```python
from build123d import *

# Parameters (mm, degrees)
F1_DEPTH = 16


with BuildPart() as f1:
    # F0 (on Top) → F1 (new body)
    with BuildSketch(Plane.XY):
        Polygon((0.414211, 0.041402), (-1.415181, 0.041402), (-1.411876, 0), (-0.781621, 0), (-0.497795, -0.270558), (0.132981, -0.270558), (0.417517, 0), align=None)
        Polygon((0.420945, 0.041402), (0.414211, 0.041402), (0.417517, 0), align=None)
        Polygon((2.243604, 0.041402), (0.420945, 0.041402), (0.417517, 0), (1.047772, 0), (1.331597, -0.270558), (1.962374, -0.270558), (2.246909, 0), align=None)
        Polygon((2.250337, 0.041402), (2.243604, 0.041402), (2.246909, 0), align=None)
        Polygon((4.072996, 0.041402), (2.250337, 0.041402), (2.246909, 0), (2.877164, 0), (3.160989, -0.270558), (3.791766, -0.270558), (4.076301, 0), align=None)
        Polygon((4.079729, 0.041402), (4.072996, 0.041402), (4.076301, 0), align=None)
        Polygon((5.902388, 0.041402), (4.079729, 0.041402), (4.076301, 0), (4.706556, 0), (4.990381, -0.270558), (5.621158, -0.270558), (5.905694, 0), align=None)
        Polygon((5.909122, 0.041402), (5.902388, 0.041402), (5.905694, 0), align=None)
        Polygon((7.73178, 0.041402), (5.909122, 0.041402), (5.905694, 0), (6.535948, 0), (6.819774, -0.270558), (7.450551, -0.270558), (7.735086, 0), align=None)
        Polygon((7.738514, 0.041402), (7.73178, 0.041402), (7.735086, 0), align=None)
        Polygon((9.561173, 0.041402), (7.738514, 0.041402), (7.735086, 0), (8.365341, 0), (8.649166, -0.270558), (9.279943, -0.270558), (9.564478, 0), align=None)
        Polygon((9.567906, 0.041402), (9.561173, 0.041402), (9.564478, 0), align=None)
        Polygon((11.390565, 0.041402), (9.567906, 0.041402), (9.564478, 0), (10.194733, 0), (10.478558, -0.270558), (11.109335, -0.270558), (11.39387, 0), align=None)
        Polygon((11.397298, 0.041402), (11.390565, 0.041402), (11.39387, 0), align=None)
        Polygon((13.219957, 0.041402), (11.397298, 0.041402), (11.39387, 0), (12.024125, 0), (12.307951, -0.270558), (12.938727, -0.270558), (13.223263, 0), align=None)
        Polygon((13.226691, 0.041402), (13.219957, 0.041402), (13.223263, 0), align=None)
        Polygon((15.04935, 0.041402), (13.226691, 0.041402), (13.223263, 0), (13.853518, 0), (14.137343, -0.270558), (14.76812, -0.270558), (15.052655, 0), align=None)
        Polygon((15.056083, 0.041402), (15.04935, 0.041402), (15.052655, 0), align=None)
        Polygon((16.878742, 0.041402), (15.056083, 0.041402), (15.052655, 0), (15.68291, 0), (15.966735, -0.270558), (16.597512, -0.270558), (16.882047, 0), align=None)
        Polygon((16.885475, 0.041402), (16.878742, 0.041402), (16.882047, 0), align=None)
        Polygon((18.708134, 0.041402), (16.885475, 0.041402), (16.882047, 0), (17.512302, 0), (17.796127, -0.270558), (18.426904, -0.270558), (18.711439, 0), align=None)
        Polygon((18.714868, 0.041402), (18.708134, 0.041402), (18.711439, 0), align=None)
        Polygon((20.537526, 0.041402), (18.714868, 0.041402), (18.711439, 0), (19.341694, 0), (19.62552, -0.270558), (20.256296, -0.270558), (20.540832, 0), align=None)
        Polygon((20.54426, 0.041402), (20.537526, 0.041402), (20.540832, 0), align=None)
        Polygon((22.366919, 0.041402), (20.54426, 0.041402), (20.540832, 0), (21.171087, 0), (21.454912, -0.270558), (22.085689, -0.270558), (22.370224, 0), align=None)
        Polygon((22.373652, 0.041402), (22.366919, 0.041402), (22.370224, 0), align=None)
        Polygon((24.196311, 0.041402), (22.373652, 0.041402), (22.370224, 0), (23.000479, 0), (23.284304, -0.270558), (23.915081, -0.270558), (24.199616, 0), align=None)
        Polygon((24.203044, 0.041402), (24.196311, 0.041402), (24.199616, 0), align=None)
        Polygon((26.025703, 0.041402), (24.203044, 0.041402), (24.199616, 0), (24.829871, 0), (25.113696, -0.270558), (25.744473, -0.270558), (26.029009, 0), align=None)
        Polygon((26.032437, 0.041402), (26.025703, 0.041402), (26.029009, 0), align=None)
        Polygon((27.855095, 0.041402), (26.032437, 0.041402), (26.029009, 0), (26.659264, 0), (26.943089, -0.270558), (27.573866, -0.270558), (27.858401, 0), align=None)
        Polygon((27.861829, 0.041402), (27.855095, 0.041402), (27.858401, 0), align=None)
        Polygon((29.684488, 0.041402), (27.861829, 0.041402), (27.858401, 0), (28.488656, 0), (28.772481, -0.270558), (29.403258, -0.270558), (29.687793, 0), align=None)
        Polygon((29.691221, 0.041402), (29.684488, 0.041402), (29.687793, 0), align=None)
        Polygon((31.51388, 0.041402), (29.691221, 0.041402), (29.687793, 0), (30.318048, 0), (30.601873, -0.270558), (31.23265, -0.270558), (31.517185, 0), align=None)
        Polygon((31.520614, 0.041402), (31.51388, 0.041402), (31.517185, 0), align=None)
        Polygon((33.3467, 0.041402), (31.520614, 0.041402), (31.517185, 0), (32.14744, 0), (32.431266, -0.270558), (33.062042, -0.270558), (33.346578, 0), (33.348323, 0.021078), align=None)
        Polygon((33.350006, 0.041402), (33.3467, 0.041402), (33.348323, 0.021078), align=None)
        Polygon((35.176093, 0.041402), (33.350006, 0.041402), (33.348323, 0.021078), (33.350006, 0), (33.980261, 0), (34.264086, -0.270558), (34.894863, -0.270558), (35.179398, 0), align=None)
        Polygon((35.182826, 0.041402), (35.176093, 0.041402), (35.179398, 0), align=None)
        Polygon((37.005485, 0.041402), (35.182826, 0.041402), (35.179398, 0), (35.809653, 0), (36.093478, -0.270558), (36.724255, -0.270558), (37.00879, 0), align=None)
        Polygon((37.012218, 0.041402), (37.005485, 0.041402), (37.00879, 0), align=None)
        Polygon((38.841611, 0.041402), (37.012218, 0.041402), (37.00879, 0), (37.639045, 0), (37.922871, -0.270558), (38.553647, -0.270558), (38.838183, 0), align=None)
    extrude(amount=F1_DEPTH)


solid = f1.part
```
Part model, mm, in its own coordinate system. Give positions to 0.01 mm unless a question says otherwise; leave off trailing zeros. Use a Markdown table: item, result. Add a question column.
(1) Saw through at A-A, the plane y = -0.1. Give the number of separate pieces and of enclosed holes in the cut face, and give its area (3 significant figures).
(2) Drop flat-ended pins along their axis: P1, Ø0.5, axis at x = 37, z = 10, coming from the -Y side; P2, Ø0.7, axis at x = 8, z = 11, coming from the -Y side; P3, Ø0.5, axis at x = 4.5, z = 8, coming from the -Y side; P4, Ø5, axis at x = 6, z = 13, coming from the -Y side. Give the stop position or say it passes through.
(3) Probe line 1 along Y through (x, z) = (24, 4.25). List the from-to ranges inside material, lowest first. Write a range as [from, to].
Answer key:
| question | item | result |
|---|---|---|
| 1 | separate pieces | 22 |
| 1 | enclosed holes | 0 |
| 1 | area | 348 mm^2 |
| 2 | P1 | y = -0.25 |
| 2 | P2 | y = -0.08 |
| 2 | P3 | y = -0.04 |
| 2 | P4 | y = -0.27 |
| 3 | line 1 | [-0.19, 0.04] |
